Could you check a few things on this model? Use its own coordinates, in mm. Face numbers are marked on the shaded views. A direction names the side the tool comes from. Coordinates: 2 decimals unless noted, no trailing zeros. Order: outer loops, then holes, each group sorted by start corner. A loop starts at its lowest first (then second) coordinate and runs counter-clockwise, first axis right, second up. Notation, with made-up numbers: (7, 33.5) - (62, 33.5) arc R26 cw to (62, 60.5) - close; hole circle Ø9 at (23, 18). An arc over 180 degrees is marked (long way). One line per item, written item: value.
from build123d import *

# Parameters (mm, degrees)
F1_DEPTH = 203.2
F2_DEPTH = 6.35
F4_DEPTH = 6.35
F5_W     = 19.05
F5_H     = 278.024951
F5_W_2   = 209.55
F5_H_2   = 12.7
F5_H_3   = 278.110252
F6_DEPTH = 6.35


with BuildPart() as f1:
    # F0 (on Right) → F1 (new body)
    with BuildSketch(Plane.YZ):
        Polygon((0, 6.35), (-11.581397, 6.35), (-289.534933, 158.75), (-289.534933, 151.508147), (-13.207997, 0), (0, 0), align=None)
    extrude(amount=F1_DEPTH)

    # F0 (on Right) → F2 (join)
    with BuildSketch(Plane.YZ):
        Polygon((-13.207997, 0), (-289.534933, 151.508147), (-289.534933, 0), align=None)
    extrude(amount=F2_DEPTH)

    # F3 (on face) → F4 (join)
    with BuildSketch(Plane.YZ.offset(203.2)):
        Polygon((-11.581397, 6.35), (-289.534933, 158.75), (-289.534933, 0), (0, 0), (0, 6.35), align=None)
    extrude(amount=F4_DEPTH)

    # F5 (on Top) → F6 (join)
    with BuildSketch(Plane.XY):
        with Locations((-9.525, -150.547525)):
            Rectangle(F5_W, F5_H)
        with Locations((104.775, 6.35)):
            Rectangle(F5_W_2, F5_H_2)
        with Locations((219.075, -150.504874)):
            Rectangle(F5_W, F5_H_3)
    extrude(amount=F6_DEPTH)


solid = f1.part
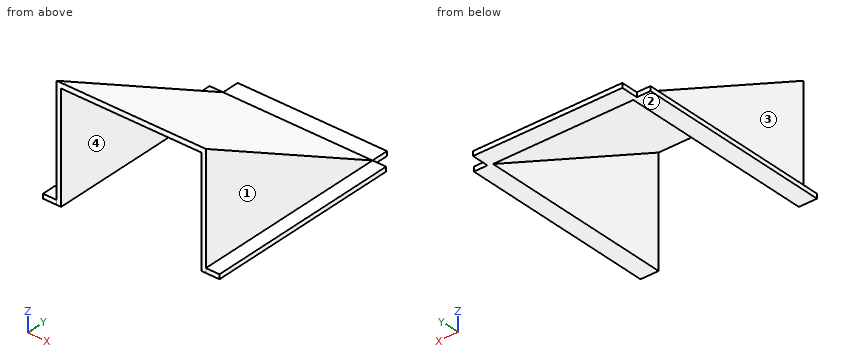
Item 1: I want a section at C-C on z = 114.5. Please give me the cut outline in (x, y), then the cut area to 3 significant figures.
Conclusion:
outline: (0, -289.53) - (6.35, -289.53) - (6.35, -222.04) - (203.2, -222.04) - (203.2, -289.53) - (209.55, -289.53) - (209.55, -208.83) - (0, -208.83) - close
area: 3,620 mm²
Item 2: I want a section at D-D on y = -197. Please give me the cut outline in (x, z), then the cut area to 3 significant figures.
Conclusion:
outline: (-19.05, 0) - (6.35, 0) - (6.35, 100.77) - (203.2, 100.77) - (203.2, 0) - (228.6, 0) - (228.6, 6.35) - (209.55, 6.35) - (209.55, 108.01) - (0, 108.01) - (0, 6.35) - (-19.05, 6.35) - close
area: 3,040 mm²
Item 3: I want a section at B-B on y = -97. Please give me the cut outline in (x, z).
Conclusion:
outline: (-19.05, 0) - (6.35, 0) - (6.35, 45.94) - (203.2, 45.94) - (203.2, 0) - (228.6, 0) - (228.6, 6.35) - (209.55, 6.35) - (209.55, 53.18) - (0, 53.18) - (0, 6.35) - (-19.05, 6.35) - close
Item 4: If I drill on probe 1 along X at (y, z) = (-155.5, 39.5); probe 2 along X at (y, z) = (-152, 81.5); probe 3 along Z at (x, y) = (63, -9), over which ranges is the centre line in solid material (lowest first)?
Conclusion:
probe 1: 0 to 6.35, 203.2 to 209.55
probe 2: 0 to 209.55
probe 3: 0 to 6.35
Item 5: I'm going to push flat-ended pins straight in: pin 1 Ø1.9 at (y, z) = (6.5, 4.5) entering from +X; pin 2 Ø4 at (y, z) = (-240.5, 75) entering from -X; pin 3 Ø5 at (x, z) = (-10.5, 3.5) entering from +Y. Where does each tip first touch, or does it pass through?
Conclusion:
pin 1: x = 209.55
pin 2: x = 0
pin 3: y = -11.54
Item 6: For the marked faces 1, 2, 3 and 4, which set-ups out of +Z, -Z, +X, -X, +Y, -Y let a thin tool reach every point of the face, with its end or its side?
Conclusion:
face 1: +Z, +X, +Y, -Y
face 2: -Z, +X, -X, +Y, -Y
face 3: +Z, -X, +Y, -Y
face 4: -Z, -Y
Item 7: I want a section at A-A on x = 91.5. Please give me the cut outline in (y, z).
Conclusion:
outline: (-289.53, 151.51) - (-13.21, 0) - (12.7, 0) - (12.7, 6.35) - (-11.58, 6.35) - (-289.53, 158.75) - close
